Build history of the part. All positions in model axes, mm. A direction names the side the tool comes from. Round coordinates to 2 decimals unless told otherwise and drop trailing zeros. Loops run counter-clockwise (first coordinate to the right, second up) from the corner with the lowest first, then second, coordinate; pieces in that order, holes last. Notation, with made-up numbers: (-30, 74) - (3, 74) arc R21 cw to (3, 112) - close; hole circle Ø10 at (25.25, 50.5). An arc over 180 degrees is marked (long way). Use a Markdown table: item, result.
from build123d import *

# Parameters (mm, degrees)
ESQUISSE1_W             = 20
ESQUISSE1_H             = 40
BOSS_EXTRU_1_DEPTH      = 5
ESQUISSE5_R             = 8
ENL_V_MAT_EXTRU_2_DEPTH = 5
ENL_V_MAT_EXTRU_3_DEPTH = 46
CHANFREIN1_SIZE         = 0.5


with BuildPart() as part:
    # Esquisse1 → Boss.-Extru.1 (new body)
    with BuildSketch(Plane.XY):
        with Locations((10, 20)):
            Rectangle(ESQUISSE1_W, ESQUISSE1_H)
    extrude(amount=BOSS_EXTRU_1_DEPTH)

    # Esquisse5 → Enlèv. mat.-Extru.2 (cut)
    with BuildSketch(Plane.XY.offset(5)):
        with Locations((10, 20)):
            Circle(ESQUISSE5_R)
    extrude(amount=-ENL_V_MAT_EXTRU_2_DEPTH, mode=Mode.SUBTRACT)

    # Esquisse6 → Enlèv. mat.-Extru.3 (cut, through all)
    with BuildSketch(Plane.XY.offset(5)):
        with BuildLine():
            Line((7.5, 38), (12.5, 38))
            ThreePointArc((12.5, 38), (15.5, 35), (12.5, 32))
            Line((12.5, 32), (7.5, 32))
            ThreePointArc((7.5, 32), (4.5, 35), (7.5, 38))
        make_face()
        with BuildLine():
            Line((7.5, 2), (12.5, 2))
            ThreePointArc((12.5, 2), (15.5, 5), (12.5, 8))
            Line((12.5, 8), (7.5, 8))
            ThreePointArc((7.5, 8), (4.5, 5), (7.5, 2))
        make_face()
    extrude(amount=-ENL_V_MAT_EXTRU_3_DEPTH, mode=Mode.SUBTRACT)

    # Chanfrein1
    chanfrein1_edges = [part.edges().sort_by_distance(p)[0] for p in [
        (20, 20, 5),
        (10, 40, 5),
        (2, 20, 0),
        (2, 20, 5),
        (4.5, 35, 0),
        (10, 38, 0),
        (15.5, 35, 0),
        (10, 32, 0),
        (4.5, 35, 5),
        (10, 32, 5),
        (15.5, 35, 5),
        (10, 38, 5),
        (4.5, 5, 0),
        (10, 8, 0),
        (15.5, 5, 0),
        (10, 2, 0),
        (4.5, 5, 5),
        (10, 2, 5),
        (15.5, 5, 5),
        (10, 8, 5),
        (0, 20, 5),
        (10, 40, 0),
        (20, 20, 0),
        (0, 20, 0),
        (10, 0, 5),
        (0, 40, 2.5),
        (20, 40, 2.5),
        (0, 0, 2.5),
    ]]
    chamfer(chanfrein1_edges, length=CHANFREIN1_SIZE)


solid = part.part
Q1. Pull direction X, two halves, no side cores. Call faces 5 (the face through (4.5, 5.1, 2.5)), 6 (the face through (10, 0, 2)), 7 (the face through (0, 20, 2)): pulls with the +X half, pulls with the -X half, needs draft (parallel to the pull), parting line crosses it, or undercut.
Results found:
| item | result |
|---|---|
| face 5 | undercut |
| face 6 | needs draft |
| face 7 | pulls with the -X half |
Q2. Cut at B-B, the plane x = 10. Count the separate pieces of the cut face and the enclosed holes in it, plus the area to 3 significant figures.
Results found:
| item | result |
|---|---|
| separate pieces | 4 |
| enclosed holes | 0 |
| area | 58.1 mm2 |
Q3. Cut at D-D, the plane y = 35. List the corners of the cut face in (x, z), plus the area to 3 significant figures.
Results found:
| item | result |
|---|---|
| outline | (0, 0.5) - (0.5, 0) - (4, 0) - (4.5, 0.5) - (4.5, 4.5) - (4, 5) - (0.5, 5) - (0, 4.5) - close; (15.5, 0.5) - (16, 0) - (19.5, 0) - (20, 0.5) - (20, 4.5) - (19.5, 5) - (16, 5) - (15.5, 4.5) - close |
| area | 44.0 mm2 |
Q4. Cut at C-C, the plane z = 3. List the corners of the cut face in (x, y).
Results found:
| item | result |
|---|---|
| outline | (0, 0.5) - (0.5, 0) - (20, 0) - (20, 39.5) - (19.5, 40) - (0.5, 40) - (0, 39.5) - close; hole circle Ø16 at (10, 20); hole (7.5, 2) - (12.5, 2) arc R3 ccw to (12.5, 8) - (7.5, 8) arc R3 ccw to start; hole (7.5, 32) - (12.5, 32) arc R3 ccw to (12.5, 38) - (7.5, 38) arc R3 ccw to start |
Q5. Probe line 1 (Y direction, x = 10, z = 2.35); line 2 (Y direction, x = 5, z = 4.75); line 3 (Y direction, x = 3.75, z = 0.9). List the from-to ranges inside material, lowest first.
Results found:
| item | result |
|---|---|
| line 1 | y = 0 to 2, 8 to 12, 28 to 32, 38 to 40 |
| line 2 | y = 0.25 to 2.92, 7.08 to 13.44, 26.56 to 32.92, 37.08 to 39.75 |
| line 3 | y = 0 to 15.01, 24.99 to 40 |
Q6. Cut at A-A, the plane y = 20. List the corners of the cut face in (x, z), plus the area to 3 significant figures.
Results found:
| item | result |
|---|---|
| outline | (0, 0.5) - (0.5, 0) - (1.5, 0) - (2, 0.5) - (2, 4.5) - (1.5, 5) - (0.5, 5) - (0, 4.5) - close; (18, 0.5) - (18.5, 0) - (19.5, 0) - (20, 0.5) - (20, 4.5) - (19.5, 5) - (18.5, 5) - (18, 4.5) - close |
| area | 19.0 mm2 |
Q7. Which spindle directions (+Z, -Z, +X, -X, +Y, -Y) get a long thin tool onto all of the face, cutting with end or side? Do faces 1 (the face through (4.365, 35.069, 0.365)), 2 (the face through (10, 40, 2)), 3 (the face through (4.5, 34.9, 2.5)), 4 (the face through (15.635, 4.931, 4.635)). Say none if no direction does.
Results found:
| item | result |
|---|---|
| face 1 | -Z |
| face 2 | +Z, -Z, +X, -X, +Y |
| face 3 | +Z, -Z |
| face 4 | +Z |
